from build123d import *

# Parameters (mm, degrees)
F2_W     = 95
F2_H     = 89
F0_W     = 95
F0_H     = 77
F7_R     = 37
F8_DEPTH = 85.8
F9_R     = 4


# Not quite as in the source:
# - a feature names something its author has since deleted; it is built from what else it names


with BuildPart() as f3:
    # F2 (on offset) → F3 section 0
    with BuildSketch(Plane.XY.offset(70)):
        with Locations((-47.5, -38.5)):
            Rectangle(F2_W, F2_H)
    # F0 (on Top) → F3 section 1
    with BuildSketch(Plane.XY):
        with Locations((-47.5, -38.5)):
            Rectangle(F0_W, F0_H)
    loft()

    # F7 (on face) → F8 (cut)
    with BuildSketch(Plane(origin=(-27.2627936506, 0, 102.6103478024), x_dir=(0.966468953, 0, 0.2567834941), z_dir=(-0.2567834941, 0, 0.966468953))):
        with Locations((-34.7436182201, -38.5)):
            Circle(F7_R)
    extrude(amount=-F8_DEPTH, mode=Mode.SUBTRACT)

    # F9
    f9_edges = [f3.edges().sort_by_distance(p)[0] for p in [
        (-47.5, -77, 0),
        (0, -38.5, 0),
        (-47.5, 0, 0),
        (0, -80, 35),
        (0, 3, 35),
    ]]
    fillet(f9_edges, radius=F9_R)


solid = f3.part
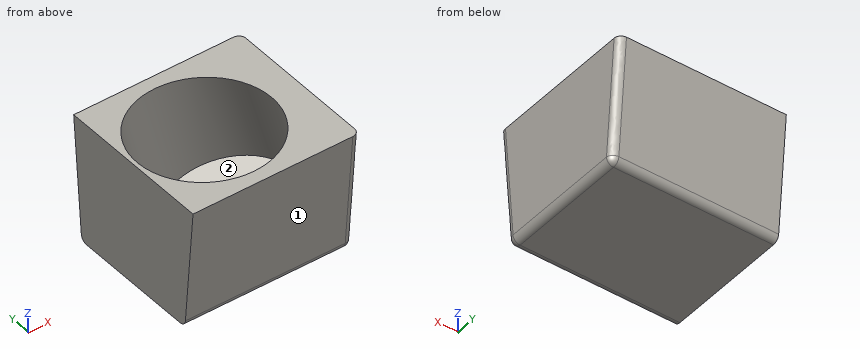
Verification items for the finished model (mm, model axes). Face numbers are marked on the shaded views. Coordinates: 2 decimals unless noted, no trailing zeros. One line per item, written item: value.
1. Gauge pin test, flat ends, axial feed: P1, Ø3, axis at y = -66, z = 7.5, coming from the +X side; P2, Ø8, axis at x = -70, z = 41.5, coming from the -Y side; P3, Ø3, axis at x = -79, z = 15.5, coming from the +Y side. Record the tip position at first contact, or that the pin passes through.
Answers follow:
P1: x = 0
P2: y = -80.9
P3: y = 1.46
2. Mould release check, pull along X, two halves, no side actions. Record for the marked faces 1 and 2: pulls with the +X half, pulls with the -X half, needs draft (parallel to the pull), parting line crosses it, or undercut.
Answers follow:
face 1: needs draft
face 2: undercut
3. Material ranges on line 1 along Y through (x, z) = (-63.5, 12.5); line 2 along Y through (x, z) = (-71.5, 13.5); line 3 along X through (y, z) = (-16.5, 31), recorded low to high. Write a range as from..to.
Answers follow:
line 1: -78.07..-67.15, -9.85..1.07
line 2: -78.16..-58.86, -18.14..1.16
line 3: -95..-74.97, -13.4..0
